Check sheet for the drawn part. Datum: minimum x, y, z corner. Units: mm. A direction names the side the tool comes from. Coordinates: 2 decimals unless noted, no trailing zeros. Loops run counter-clockwise (first coordinate to the right, second up) from the corner with the lowest first, then second, coordinate; pieces in that order, holes last. Notation, with made-up numbers: (54, -37) - (101, -37) arc R18 cw to (101, -27) - close; hole circle Ø2 at (61.25, -21.75). An arc over 180 degrees is marked (long way). Write item = value, one per line. Start each with the question number.
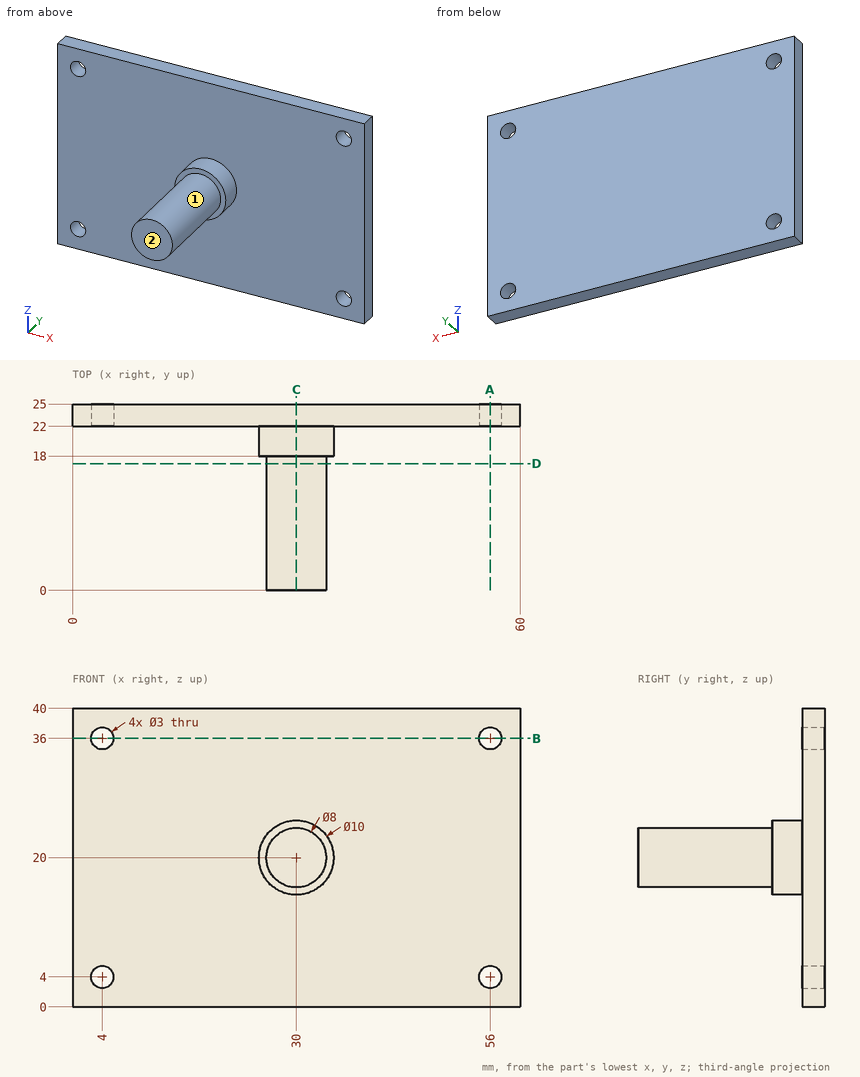
(1) Sectioned sample at C-C on x = 30. Enter the section's corners in (y, z).
(2) Depth check by flat-ended pin: pin 1 (4 mm diameter, centred on y = 16.5, z = 21.5, fed in from +X); pin 2 (3 mm diameter, centred on x = 27.5, z = 19, fed in from -Y); pin 3 (12 mm diameter, centred on x = 41.5, z = 6, fed in from -Y); pin 4 (4 mm diameter, centred on x = 31, y = 11, fed in from -Z). Enter the tip coordinate at first touch or a pass-through.
(3) Sectioned sample at A-A on x = 56. Enter the section's corners in (y, z), plus the area to 3 significant figures.
(4) Sectioned sample at D-D on y = 17. Enter the section's corners in (x, z).
(5) Tool access check on the marked faces 1 and 2. Record the directions out of +Z, -Z, +X, -X, +Y, -Y that give a thin tool (end or side, any length) a straight path to the whole face; none if there is none.
(6) Scan lines: line 1 (X direction, y = 23.8, z = 36); line 2 (Y direction, x = 46.5, z = 22.5); line 3 (Z direction, x = 31, y = 5.75). Record each from-to range of solid material in increasing order.
(7) Sectioned sample at B-B on z = 36. Enter the section's corners in (x, y).
Working result:
q1.outline = (0, 16) - (18, 16) - (18, 15) - (22, 15) - (22, 0) - (25, 0) - (25, 40) - (22, 40) - (22, 25) - (18, 25) - (18, 24) - (0, 24) - close
q2.pin_1 = 35
q2.pin_2 = 0
q2.pin_3 = 22
q2.pin_4 = 16
q3.outline = (22, 0) - (25, 0) - (25, 2.5) - (22, 2.5) - close; (22, 5.5) - (25, 5.5) - (25, 34.5) - (22, 34.5) - close; (22, 37.5) - (25, 37.5) - (25, 40) - (22, 40) - close
q3.area = 102 mm2
q4.outline = circle Ø8 at (30, 20)
q5.face_1 = -Y
q5.face_2 = +Z, -Z, +X, -X, -Y
q6.line_1 = 0 to 2.5, 5.5 to 54.5, 57.5 to 60
q6.line_2 = 22 to 25
q6.line_3 = 16.13 to 23.87
q7.outline = (0, 22) - (2.5, 22) - (2.5, 25) - (0, 25) - close; (5.5, 22) - (54.5, 22) - (54.5, 25) - (5.5, 25) - close; (57.5, 22) - (60, 22) - (60, 25) - (57.5, 25) - close
